Source: CAD feature listing. Evaluate the final solid. Frame: model axes, mm. Face numbers are marked on the shaded views. A direction names the side the tool comes from. Give positions to 0.01 mm unless a question says otherwise; leave off trailing zeros. Order: outer loops, then holes, each group sorted by start corner. A loop starts at its lowest first (then second) coordinate and runs counter-clockwise, first axis right, second up. Notation, with made-up numbers: M -5.75,-26 L 16.25,-26 A26 ccw 16.25,-11 Z; hole C -7,-22.5 d4. An arc over 180 degrees is marked long. Answer in a Markdown table with one row per item. Add a question column.
(1) Pin query (flat end, axial travel): P1, Ø12.5, axis at x = 34.5, y = -7.5, coming from the +Z side; P2, Ø6, axis at x = 47, y = -0.5, coming from the +Z side. Return the tip coordinate at first contact, or that it passes through.
(2) Section query A-A, the plane z = 23. Return loops of the section in (x, y).
(3) Section query D-D, the plane x = 23. Return loops of the section in (y, z).
(4) Section query C-C, the plane z = 10. Return loops of the section in (x, y), plus the area to 3 significant figures.
(5) Material intervals for line 1 along Y through (x, z) = (52, 28.5); line 2 along X through (y, z) = (10, 25.5); line 3 along Z through (x, y) = (33, -16), sorted ascending.
(6) Section query B-B, the plane y = 22. Return loops of the section in (x, z).
(7) Mould query, pull axis X, two halves, no side actions, for the marked faces 1, 2 and 3. Classes: pulls with the +X half, pulls with the -X half, needs draft (parallel to the pull), parting line crosses it, or undercut.
(8) Set-up query: the marked faces 4 and 5. Return all of +Z, -Z, +X, -X, +Y, -Y with unobstructed straight access to the full face (end or side cutting, diameter ignored); none if empty.
from build123d import *

# Parameters (mm, degrees)
F0_R     = 9.4158486149
F1_DEPTH = 25.4
F4_DEPTH = 27.5
F5_W     = 15.7655179501
F5_H     = 7.5176365208
F6_DEPTH = 25.4


with BuildPart() as f1:
    # F0 (on Front) → F1 (new body)
    with BuildSketch(Plane.XZ):
        with BuildLine():
            Line((-26.7482474446, -27.6464950293), (26.7482474446, -27.6464950293))
            Line((26.7482474446, -27.6464950293), (26.7482474446, 27.6464950293))
            ThreePointArc((26.7482474446, 27.6464950293), (0, 0.8982475847), (-26.7482474446, 27.6464950293))
            Line((-26.7482474446, 27.6464950293), (-26.7482474446, -27.6464950293))
        make_face()
        with BuildLine():
            ThreePointArc((-26.7482474446, 27.6464950293), (0, 0.8982475847), (26.7482474446, 27.6464950293))
            ThreePointArc((26.7482474446, 27.6464950293), (0, 54.394742474), (-26.7482474446, 27.6464950293))
        make_face()
        with Locations((0, 27.6464950293)):
            Circle(F0_R, mode=Mode.SUBTRACT)
    extrude(amount=F1_DEPTH)


with BuildPart() as f4:
    # F3 (on Front) → F4 (new body, symmetric)
    with BuildSketch(Plane.XZ):
        Polygon((0, 32.1222431958), (0, 0), (56.9529347122, 0), (56.9529347122, 32.1222431958), (41.1874167621, 32.1222431958), (41.1874167621, 20.1010350138), (15.7655179501, 20.1010350138), (15.7655179501, 32.1222431958), align=None)
    extrude(amount=F4_DEPTH, both=True)

    # F5 (on face) → F6 (cut)
    with BuildSketch(Plane.XY.offset(32.1222431958)):
        with Locations((49.0701757371, 0.0409217319)):
            Rectangle(F5_W, F5_H)
    extrude(amount=-F6_DEPTH, mode=Mode.SUBTRACT)


solid = f4.part
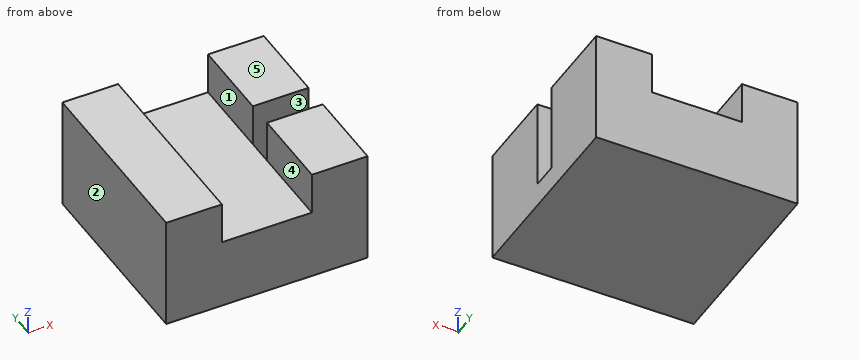
Values follow:
| question | item | result |
|---|---|---|
| 1 | P1 | stops at z = 20.1 |
| 1 | P2 | stops at z = 6.72 |
| 2 | outline | M 0,-27.5 L 15.77,-27.5 L 15.77,27.5 L 0,27.5 Z; M 41.19,-27.5 L 56.95,-27.5 L 56.95,-3.72 L 41.19,-3.72 Z; M 41.19,3.8 L 56.95,3.8 L 56.95,27.5 L 41.19,27.5 Z |
| 3 | outline | M -27.5,0 L 27.5,0 L 27.5,20.1 L -27.5,20.1 Z |
| 4 | outline | M 0,-27.5 L 56.95,-27.5 L 56.95,-3.72 L 41.19,-3.72 L 41.19,3.8 L 56.95,3.8 L 56.95,27.5 L 0,27.5 Z |
| 4 | area | 3,010 mm² |
| 5 | line 1 | y = -27.5 to -3.72, 3.8 to 27.5 |
| 5 | line 2 | x = 0 to 15.77, 41.19 to 56.95 |
| 5 | line 3 | z = 0 to 20.1 |
| 6 | outline | M 0,0 L 56.95,0 L 56.95,32.12 L 41.19,32.12 L 41.19,20.1 L 15.77,20.1 L 15.77,32.12 L 0,32.12 Z |
| 7 | face 1 | undercut |
| 7 | face 2 | pulls with the -X half |
| 7 | face 3 | needs draft |
| 8 | face 4 | +Z, +Y, -Y |
| 8 | face 5 | +Z, +X, -X, +Y, -Y |
